Part model, mm, in its own coordinate system. A direction names the side the tool comes from. Give positions to 0.01 mm unless a question says otherwise; leave off trailing zeros. Write each loop counter-clockwise with the first axis right and the second up, starting at its lowest first coordinate (ties: lowest second). Pieces come first, ordered by that corner, then holes. Notation, with made-up numbers: (73, 23.25) - (93, 23.25) arc R7 ccw to (93, 36.25) - close; hole circle Ø10 at (49, -33). An arc over 180 degrees is marked (long way). Answer in a Markdown table with one row per item. Add a question column.
1. Band-saw the part on C-C on z = 15. Write the cut outline in (x, y).
2. Band-saw the part on D-D on x = 32. Write the cut outline in (y, z).
3. Band-saw the part on B-B on y = 44. Write the cut outline in (x, z), plus the area to 3 significant figures.
4. Probe line 1 along Y through (x, z) = (43, 47); line 2 along X through (y, z) = (39, 20). List the from-to ranges inside material, lowest first.
5. Band-saw the part on A-A on x = 41.5. Write the cut outline in (y, z), plus the area to 3 significant figures.
6. Drop flat-ended pins along their axis: pin 1 Ø12 at (x, y) = (37.5, 39) entering from +Z; pin 2 Ø12 at (x, z) = (42, 17) entering from +Y; pin 3 Ø12 at (y, z) = (38.5, 15.5) entering from +X; pin 4 Ø2 at (x, z) = (21.5, 12) entering from +Y. Give the stop position or say it passes through.
7. Which spindle directions (+Z, -Z, +X, -X, +Y, -Y) get a long thin tool onto all of the face, cutting with end or side? Do faces 5 (the flat face through (40, 35, 17)), 6 (the flat face through (50, 19, 19)), 7 (the flat face through (6.5, 5.7, 35.4)), 8 (the flat face through (42, 30, 43)), 9 (the flat face through (18, 35, 30)). Say none if no direction does.
8. Pull direction X, two halves, no side cores. Call faces 1 (the flat face through (25, 6, 37)), 2 (the flat face through (30, 42, 18)), 3 (the flat face through (30, 0, 19)), 4 (the flat face through (17, 10, 30)): released by +X, released by -X, zero draft, split by the parting line, or undercut.
```python
from build123d import *

# Parameters (mm, degrees)
F0_W      = 50
F0_H      = 50
F1_DEPTH  = 50
F6_W      = 15
F6_H      = 53.66563146
F7_DEPTH  = 17.88954382
F11_W     = 15
F11_H     = 58
F12_DEPTH = 24.001
F17_DEPTH = 16.6676666667
F20_DEPTH = 8.7297156094
F23_DEPTH = 9.2317692308
F27_W     = 15
F27_H     = 15
F28_DEPTH = 20


with BuildPart() as f1:
    # F0 (on Top) → F1 (new body)
    with BuildSketch(Plane.XY):
        with Locations((25, 25)):
            Rectangle(F0_W, F0_H)
    extrude(amount=F1_DEPTH)

    # F6 (on 3pt) → F7 (cut, through all)
    with BuildSketch(Plane(origin=(0, -4, 2), x_dir=(1, 0, 0), z_dir=(0, -0.894427191, 0.4472135955))):
        with Locations((17.5, 26.83281573)):
            Rectangle(F6_W, F6_H)
    extrude(amount=F7_DEPTH, mode=Mode.SUBTRACT)

    # F11 (on 3pt) → F12 (cut, through all)
    with BuildSketch(Plane(origin=(0, 36.8, 27.6), x_dir=(-1, 0, 0), z_dir=(0, 0.8, 0.6))):
        with Locations((-17.5, -1)):
            Rectangle(F11_W, F11_H)
    extrude(amount=F12_DEPTH, mode=Mode.SUBTRACT)

    # F16 (on 3pt) → F17 (cut, through all)
    with BuildSketch(Plane(origin=(44.4444444444, 22.2222222222, 44.4444444444), x_dir=(-0.2357022604, 0.9428090416, -0.2357022604), z_dir=(0.6666666667, 0.3333333333, 0.6666666667))):
        Polygon((29.4627825494, 17.6776695297), (-23.5702260396, 0), (29.4627825494, -17.6776695297), align=None)
    extrude(amount=F17_DEPTH, mode=Mode.SUBTRACT)

    # F19 (on 3pt) → F20 (cut, through all)
    with BuildSketch(Plane(origin=(9.5238095238, -4.7619047619, 2.380952381), x_dir=(-0.4234048992, -0.8997354108, -0.1058512248), z_dir=(-0.8728715609, 0.4364357805, -0.2182178902))):
        Polygon((-5.2925612402, 7.2760687511), (-5.2925612402, 48.5071250073), (-27.5213184493, 46.0817687569), align=None)
    extrude(amount=-F20_DEPTH, mode=Mode.SUBTRACT)

    # F22 (on 3pt) → F23 (cut, through all)
    with BuildSketch(Plane(origin=(24.8520710059, 8.2840236686, 6.2130177515), x_dir=(-0.2985053847, 0.9514859136, -0.0746263462), z_dir=(0.9230769231, 0.3076923077, 0.2307692308))):
        Polygon((43.842978372, 48.5071250073), (12.3133471172, 46.0817687569), (43.842978372, 7.2760687511), align=None)
    extrude(amount=F23_DEPTH, mode=Mode.SUBTRACT)

    # F27 (on 3pt) → F28 (cut, through all)
    with BuildSketch(Plane.YZ.offset(30)):
        with Locations((42.5, 17.5)):
            Rectangle(F27_W, F27_H)
    extrude(amount=F28_DEPTH, mode=Mode.SUBTRACT)


solid = f1.part
```
Values:
| question | item | result |
|---|---|---|
| 1 | outline | (0, 0) - (8.75, 0) - (10, 2.5) - (25, 2.5) - (25, 0) - (50, 0) - (50, 35) - (30, 35) - (30, 50) - (25, 50) - (25, 46.25) - (10, 46.25) - (8.75, 50) - (0, 50) - close |
| 2 | outline | (0, 0) - (50, 0) - (50, 10) - (35, 10) - (35, 25) - (50, 25) - (50, 43) - (36, 50) - (0, 50) - close |
| 3 | outline | (0, 0) - (50, 0) - (50, 10) - (30, 10) - (30, 25) - (50, 25) - (50, 28) - (28, 50) - (25, 50) - (25, 18) - (10, 18) - (2, 50) - (0, 50) - close |
| 3 | area | 1,350 mm² |
| 4 | line 1 | y = 0 to 20 |
| 4 | line 2 | x = 0 to 30 |
| 5 | outline | (0, 0) - (50, 0) - (50, 10) - (35, 10) - (35, 25) - (50, 25) - (50, 33.5) - (17, 50) - (0, 50) - close |
| 5 | area | 2,000 mm² |
| 6 | pin 1 | stops at z = 49.71 |
| 6 | pin 2 | stops at y = 35 |
| 6 | pin 3 | stops at x = 50 |
| 6 | pin 4 | stops at y = 49.25 |
| 7 | face 5 | +X, +Y |
| 7 | face 6 | +Z, -Z, +X, +Y, -Y |
| 7 | face 7 | +Z, -Y |
| 7 | face 8 | +Z, +X, +Y |
| 7 | face 9 | +Z, +Y |
| 8 | face 1 | undercut |
| 8 | face 2 | released by +X |
| 8 | face 3 | zero draft |
| 8 | face 4 | undercut |
